Build history of the part. All positions in model axes, mm. A direction names the side the tool comes from. Round coordinates to 2 decimals unless told otherwise and drop trailing zeros. Order: outer loops, then holes, each group sorted by start corner. A loop starts at its lowest first (then second) coordinate and runs counter-clockwise, first axis right, second up. Notation, with made-up numbers: M -37,76 L -21,76 A27 cw -21,99 Z; hole C 35,-22 d8. An arc over 180 degrees is marked long. Use CSV: the item, a comma, the result in double quotes.
from build123d import *

# Parameters (mm, degrees)
EXTRUDE_1_DEPTH        = 15
SKETCH_4_W             = 130
SKETCH_4_H             = 53.153449772
CUT_EXTRUDE_1_DEPTH    = 70
SKETCH_5_W             = 4.882622246
SKETCH_5_H             = 40
EXTRUDE_2_DEPTH        = 20
SKETCH_6_R             = 2.5
CUT_EXTRUDE_2_DEPTH    = 186.212230178
FILLET_1_R             = 10
SKETCH_7_R             = 4.5
CUT_EXTRUDE_3_DEPTH    = 148.066550223
SKETCH_8_W             = 14
SKETCH_8_H             = 8
CUT_EXTRUDE_4_DEPTH    = 143.159857501
PATTERN_LINEAR_1_COUNT = 3
PATTERN_LINEAR_1_PITCH = 20


with BuildPart() as part:
    # 草图1 → 凸台-拉伸1 (new body)
    with BuildSketch(Plane(origin=(0, 0, 0), x_dir=(1, 0, 0), z_dir=(0, 1, 0))):
        Polygon((-65, 0), (65, 0), (65, 70), (30, 120), (-30, 120), (-65, 70), align=None)
    extrude(amount=EXTRUDE_1_DEPTH)

    # 草图2 → 放样1 section 0
    with BuildSketch(Plane(origin=(0, 15, 0), x_dir=(1, 0, 0), z_dir=(0, 1, 0))):
        with BuildLine():
            Line((-65, 70), (-61.723072318, 67.706150623))
            Line((-61.723072318, 67.706150623), (-28.617377754, 115))
            Line((-28.617377754, 115), (28.617377754, 115))
            Line((28.617377754, 115), (61.723072318, 67.706150623))
            Line((61.723072318, 67.706150623), (65, 70))
            Line((65, 70), (30, 120))
            Line((30, 120), (-30, 120))
            Line((-30, 120), (-65, 70))
        make_face()
    # 草图3 → 放样1 section 1
    with BuildSketch(Plane(origin=(0, 14.547694656, 2.565151075), x_dir=(1, 0, 0), z_dir=(0, 0.984807753012208, 0.17364817766693072))):
        with BuildLine():
            Line((-65, 71.541265376), (-61.723072318, 69.282264725))
            Line((-61.723072318, 69.282264725), (-28.617377754, 115.857614261))
            Line((-28.617377754, 115.857614261), (28.617377754, 115.857614261))
            Line((28.617377754, 115.857614261), (61.723072318, 69.282264725))
            Line((61.723072318, 69.282264725), (65, 71.541265376))
            Line((65, 71.541265376), (30, 120.781653026))
            Line((30, 120.781653026), (-30, 120.781653026))
            Line((-30, 120.781653026), (-65, 71.541265376))
        make_face()
    loft()

    # 草图9 → 放样2 section 0
    with BuildSketch(Plane(origin=(0, 14.547694656, 2.565151075), x_dir=(1, 0, 0), z_dir=(0, 0.9848077530122079, 0.17364817766693139))):
        with BuildLine():
            Line((-65, 71.541265376), (-61.723072318, 69.282264725))
            Line((-61.723072318, 69.282264725), (-28.617377754, 115.857614261))
            Line((-28.617377754, 115.857614261), (28.617377754, 115.857614261))
            Line((28.617377754, 115.857614261), (61.723072318, 69.282264725))
            Line((61.723072318, 69.282264725), (65, 71.541265376))
            Line((65, 71.541265376), (30, 120.781653026))
            Line((30, 120.781653026), (-30, 120.781653026))
            Line((-30, 120.781653026), (-65, 71.541265376))
        make_face()
    # 草图10 → 放样2 section 1
    with BuildSketch(Plane(origin=(0, 13.245333323, 4.820907073), x_dir=(1, 0, 0), z_dir=(0, 0.9396926207859081, 0.34202014332566943))):
        with BuildLine():
            Line((-65, 73.019543877), (-61.723072318, 70.794862522))
            Line((-61.723072318, 70.794862522), (-28.617377754, 116.662627845))
            Line((-28.617377754, 116.662627845), (28.617377754, 116.662627845))
            Line((28.617377754, 116.662627845), (61.723072318, 70.794862522))
            Line((61.723072318, 70.794862522), (65, 73.019543877))
            Line((65, 73.019543877), (30, 121.511859397))
            Line((30, 121.511859397), (-30, 121.511859397))
            Line((-30, 121.511859397), (-65, 73.019543877))
        make_face()
    loft()

    # 草图4 → 切除-拉伸1 (cut)
    with BuildSketch(Plane.XY):
        with Locations((0, 41.576724886)):
            Rectangle(SKETCH_4_W, SKETCH_4_H)
    extrude(amount=-CUT_EXTRUDE_1_DEPTH, mode=Mode.SUBTRACT)

    # 草图5 → 凸台-拉伸2 (add)
    with BuildSketch(Plane(origin=(0, 15, 0), x_dir=(1, 0, 0), z_dir=(0, 1, 0))):
        with Locations((62.558688877, 20)):
            Rectangle(SKETCH_5_W, SKETCH_5_H)
        with Locations((-62.558688877, 20)):
            Rectangle(SKETCH_5_W, SKETCH_5_H)
    extrude(amount=EXTRUDE_2_DEPTH)

    # 草图6 → 切除-拉伸2 (cut, through all)
    with BuildSketch(Plane.ZY.offset(65)):
        with Locations((-26.666666667, 25)):
            Circle(SKETCH_6_R)
        with Locations((-13.333333333, 25)):
            Circle(SKETCH_6_R)
    extrude(amount=-CUT_EXTRUDE_2_DEPTH, mode=Mode.SUBTRACT)

    # 圆角1
    fillet_1_edges = [part.edges().sort_by_distance(p)[0] for p in [
        (62.558688877, 35, 0),
        (62.558688877, 35, -40),
        (-62.558688877, 35, 0),
        (-62.558688877, 35, -40),
    ]]
    fillet(fillet_1_edges, radius=FILLET_1_R)

    # 草图7 → 切除-拉伸3 (cut, through all)
    with BuildSketch(Plane.XY):
        with Locations((-30, 7.5)):
            Circle(SKETCH_7_R)
        with Locations((30, 7.5)):
            Circle(SKETCH_7_R)
    extrude(amount=-CUT_EXTRUDE_3_DEPTH, mode=Mode.SUBTRACT)

    # 草图8 → 切除-拉伸4 (cut, through all)
    with BuildSketch(Plane(origin=(0, 15, 0), x_dir=(1, 0, 0), z_dir=(0, 1, 0))):
        with Locations((-30, 58.142993984)):
            Rectangle(SKETCH_8_W, SKETCH_8_H)
        with Locations((30, 58.142993984)):
            Rectangle(SKETCH_8_W, SKETCH_8_H)
    cut_extrude_4 = extrude(amount=-CUT_EXTRUDE_4_DEPTH, mode=Mode.SUBTRACT)

    # 阵列(线性)1: 切除-拉伸4 ×3
    with Locations(*[(0, 0, i * PATTERN_LINEAR_1_PITCH) for i in range(1, PATTERN_LINEAR_1_COUNT)]):
        add(cut_extrude_4, mode=Mode.SUBTRACT)


solid = part.part
(1) Cut at B-B, the plane x = -7.5. Give the cut face in (y, z).
Answer block:
outline,"M 0,-120 L 15,-120 L 35.52,-116.38 L 54.8,-109.36 L 53.15,-104.81 L 34.67,-111.53 L 15,-115 L 15,0 L 0,0 Z"
(2) Two-plate mould, pull along Z, no slides. Class faces 1 (the face through (62.59, 32.15, -36.99)), 2 (the face through (-62.52, 31.99, -2.85)), 3 (the face through (0.42, 25.404, -118.165)): released by +Z, released by -Z, zero draft, split by the parting line, or undercut.
Answer block:
face 1,"undercut"
face 2,"released by +Z"
face 3,"released by -Z"
(3) Cut at A-A, the plane z = -45. Give the cut face in (x, y).
Answer block:
outline,"M -65,0 L 65,0 L 65,15 L -65,15 Z; hole C -30,7.5 d9; hole C 30,7.5 d9"
(4) Wall check: line 1 (X direction, y = 7, z = -5); line 2 (Y direction, x = -30, z = -46); line 3 (X direction, y = 8, z = -97.5). Give the ranges that are in metal, low to high. Write a range as from..to.
Answer block:
line 1,"x = -65..-34.47, -25.53..25.53, 34.47..65"
line 2,"y = 0..3, 12..15"
line 3,"x = -45.75..-34.47, -25.53..25.53, 34.47..45.75"
(5) Drop flat-ended pins along their axis: pin 1 (2.5 mm diameter, centred on x = -63.5, y = 20.5, fed in from -Z); pin 2 (8 mm diameter, centred on x = 33, z = -41.5, fed in from +Y); pin 3 (5 mm diameter, centred on x = -50.5, y = 29.5, fed in from +Z); pin 4 (4 mm diameter, centred on y = 25, z = -26.67, fed in from -X). Give the stop position or say it passes through.
Answer block:
pin 1,"stops at z = -72.97"
pin 2,"stops at y = 15"
pin 3,"stops at z = -77.35"
pin 4,"passes through"
(6) Tool access for faces 4 (the face through (-63, 20, -40)), 5 (the face through (-0.4, 44.04, -108.12)), 6 (the face through (-25.708, 8.852, -90.666)), 7 (the face through (-23, 8, -58)): list every direction of +Z, -Z, +X, -X, +Y, -Y with a clear straight run to the whole face (end or side of a thin tool).
Answer block:
face 4,"+X, -X, +Y"
face 5,"+Z"
face 6,"+Z, -Z"
face 7,"+Y, -Y"
(7) Cut at C-C, the plane y = 7.5. Count the separate pieces of the cut face and the enclosed holes in it, and give its area (3 significant figures).
Answer block:
separate pieces,"3"
enclosed holes,"0"
area,"11,500 mm²"
